Geometry: final body of the model. Coordinates: model frame, mm. A direction names the side the tool comes from. Give positions to 0.01 mm unless a question says otherwise; leave off trailing zeros. Loops run counter-clockwise (first coordinate to the right, second up) from the corner with the lowest first, then second, coordinate; pieces in that order, holes last.
```python
from build123d import *

# Parameters (mm, degrees)
SKETCH2_W           = 11.43
SKETCH2_H           = 8.89
SKETCH2_R           = 0.445
BOSS_EXTRUDE1_DEPTH = 0.8128
SKETCH4_R           = 0.445
BOSS_EXTRUDE2_DEPTH = 0.8128


with BuildPart() as part:
    # Sketch2 → Boss-Extrude1 (new body)
    with BuildSketch(Plane.XY):
        with Locations((0, 0.635)):
            Rectangle(SKETCH2_W, SKETCH2_H)
        with Locations((-3.9243, 0.508)):
            Circle(SKETCH2_R, mode=Mode.SUBTRACT)
        with Locations((3.9243, 0.508)):
            Circle(SKETCH2_R, mode=Mode.SUBTRACT)
    extrude(amount=BOSS_EXTRUDE1_DEPTH)

    # Sketch4 → Boss-Extrude2 (add)
    with BuildSketch(Plane.XY):
        with BuildLine():
            Line((8.382, 7.874), (-8.382, 7.874))
            Line((-8.382, 7.874), (-8.382, 3.49192268))
            ThreePointArc((-8.382, 3.49192268), (-6.718325299, 2.086822944), (-6.096, 0))
            Line((-6.096, 0), (-6.096, -3.81))
            Line((-6.096, -3.81), (6.096, -3.81))
            Line((6.096, -3.81), (6.096, 0))
            ThreePointArc((6.096, 0), (6.718325299, 2.086822944), (8.382, 3.49192268))
            Line((8.382, 3.49192268), (8.382, 7.874))
        make_face()
        with Locations((-3.9243, 0.508)):
            Circle(SKETCH4_R, mode=Mode.SUBTRACT)
        with Locations((3.9243, 0.508)):
            Circle(SKETCH4_R, mode=Mode.SUBTRACT)
    extrude(amount=BOSS_EXTRUDE2_DEPTH)


solid = part.part
```
Q1. Mould query, pull axis X, two halves, no side actions, for faces 1 (the face through (6.096, -1.9, 0.4)), 2 (the face through (0.1, 7.874, 0.4)), 3 (the face through (-4.25, 0.81, 0.4)). Classes: +X half, -X half, draft (parallel to the pull), parting line (faces both ways), or undercut.
Q2. Reachability of faces 4 (the face through (-8.382, 5.7, 0.4)), 5 (the face through (-6.096, -1.9, 0.4)) from +Z, -Z, +X, -X, +Y, -Y: full face, straight path, thin tool, end or side. Return the list, or none.
Q3. Material intervals for probe 1 along X at (y, z) = (-3, 0.3); probe 2 along Y at (x, z) = (-3.75, 0.3); probe 3 along Y at (x, z) = (-6.75, 0.35), sorted ascending.
Q4. Section query B-B, the plane z = 0.2. Return loops of the section in (x, y) (3 decimals), and give its area (3 significant figures).
Q5. Section query C-C, the plane y = -2.5. Return loops of the section in (x, z).
Q6. Section query A-A, the plane x = 3.75. Return loops of the section in (y, z).
Q7. Section query D-D, the plane y = 1.5. Return loops of the section in (x, z), and give its area (3 significant figures).
Resolved:
1. face 1: +X half
1. face 2: draft
1. face 3: undercut
2. face 4: +Z, -Z, -X, +Y, -Y
2. face 5: +Z, -Z, -X, -Y
3. probe 1: x = -6.1 to 6.1
3. probe 2: y = -3.81 to 0.1, 0.92 to 7.87
3. probe 3: y = 2.13 to 7.87
4. outline: (-8.382, 3.492) arc R3.81 cw to (-6.096, 0) - (-6.096, -3.81) - (6.096, -3.81) - (6.096, 0) arc R3.81 cw to (8.382, 3.492) - (8.382, 7.874) - (-8.382, 7.874) - close; hole circle Ø0.89 at (-3.924, 0.508); hole circle Ø0.89 at (3.924, 0.508)
4. area: 166 mm2
5. outline: (-6.1, 0) - (6.1, 0) - (6.1, 0.81) - (-6.1, 0.81) - close
6. outline: (-3.81, 0) - (0.1, 0) - (0.1, 0.81) - (-3.81, 0.81) - close; (0.92, 0) - (7.87, 0) - (7.87, 0.81) - (0.92, 0.81) - close
7. outline: (-6.4, 0) - (6.4, 0) - (6.4, 0.81) - (-6.4, 0.81) - close
7. area: 10.4 mm2
